```python
from build123d import *

# Parameters (mm, degrees)
SKETCH_1_R               = 4.9
EXTRUDE_1_DEPTH          = 1.5
SKETCH_3_R               = 3.9
EXTRUDE_2_DEPTH          = 3
SKETCH_4_R               = 4.9
EXTRUDE_3_DEPTH          = 1.3
CUT_EXTRUDE_1_DEPTH      = 10.036592278
CUT_EXTRUDE_1_DEPTH_BACK = 10.036592278
SKETCH_6_R               = 0.5
CUT_EXTRUDE_2_DEPTH      = 10.036592278


with BuildPart() as part:
    # Эскиз1 → Бобышка-Вытянуть1 (new body)
    with BuildSketch(Plane.XY):
        Circle(SKETCH_1_R)
    extrude(amount=EXTRUDE_1_DEPTH)

    # Эскиз3 → Бобышка-Вытянуть2 (add)
    with BuildSketch(Plane.XY.offset(1.5)):
        Circle(SKETCH_3_R)
    extrude(amount=EXTRUDE_2_DEPTH)

    # Эскиз4 → Бобышка-Вытянуть3 (add)
    with BuildSketch(Plane.XY.offset(4.5)):
        Circle(SKETCH_4_R)
    extrude(amount=EXTRUDE_3_DEPTH)

    # Эскиз5 → Вырез-Вытянуть1 (cut, two sides: drawn at the far end of the back side and taken through both)
    with BuildSketch(Plane(origin=(0, 0, 0), x_dir=(1, 0, 0), z_dir=(0, 1, 0)).offset(-CUT_EXTRUDE_1_DEPTH_BACK)):
        Polygon((1.45, 0), (0.971990262, -0.75), (-0.971990262, -0.75), (-1.45, 0), (-1.45, 0.521018793), (1.45, 0.521018793), align=None)
    extrude(amount=CUT_EXTRUDE_1_DEPTH + CUT_EXTRUDE_1_DEPTH_BACK, mode=Mode.SUBTRACT)

    # Эскиз6 → Вырез-Вытянуть2 (cut, through all)
    with BuildSketch(Plane.XY.offset(5.8)):
        with Locations((-4.9, 0)):
            Circle(SKETCH_6_R)
        with Locations((4.9, 0)):
            Circle(SKETCH_6_R)
    extrude(amount=-CUT_EXTRUDE_2_DEPTH, mode=Mode.SUBTRACT)


solid = part.part
```
Source: CAD feature listing. Evaluate the final solid. Frame: model axes, mm. A direction names the side the tool comes from. Round coordinates to 2 decimals unless told otherwise and drop trailing zeros. Loops run counter-clockwise (first coordinate to the right, second up) from the corner with the lowest first, then second, coordinate; pieces in that order, holes last.
(1) Material intervals for probe 1 along Z at (x, y) = (4, 0.5); probe 2 along Z at (x, y) = (0.5, -4); probe 3 along X at (y, z) = (3.75, 0.7), sorted ascending.
From the geometry:
probe 1: z = 0 to 1.5, 4.5 to 5.8
probe 2: z = 0.75 to 1.5, 4.5 to 5.8
probe 3: x = -3.15 to -1, 1 to 3.15
(2) Section query C-C (z = 0.4). Output: boundary loops of the cut face in (x, y), and give its area (3 significant figures).
From the geometry:
outline: (-4.87, -0.5) arc R4.9 ccw to (-1.2, -4.75) - (-1.2, 4.75) arc R4.9 ccw to (-4.87, 0.5) arc R0.5 cw to start; (1.2, -4.75) arc R4.9 ccw to (4.87, -0.5) arc R0.5 cw to (4.87, 0.5) arc R4.9 ccw to (1.2, 4.75) - close
area: 51.5 mm2
(3) Section query A-A (x = 0). Output: boundary loops of the cut face in (y, z), and give its area (3 significant figures).
From the geometry:
outline: (-4.9, 0.75) - (4.9, 0.75) - (4.9, 1.5) - (3.9, 1.5) - (3.9, 4.5) - (4.9, 4.5) - (4.9, 5.8) - (-4.9, 5.8) - (-4.9, 4.5) - (-3.9, 4.5) - (-3.9, 1.5) - (-4.9, 1.5) - close
area: 43.5 mm2
(4) Access query for faces 1 (the flat face through (0, 0, 0.75)), 2 (the flat face through (-4, -1, 4.5)), 3 (the cylindrical face through (-4.4, 0, 0.8)). Directions: +Z, -Z, +X, -X, +Y, -Y. A direction counts if a zero-diameter tool reaches every point of the face in a straight line with its end or side. Return the directions, or none.
From the geometry:
face 1: -Z, +Y, -Y
face 2: none
face 3: +Z, -Z, -X
(5) Pull-direction query (Z, two-part tool) for faces 4 (the flat face through (3, 0, 0)), 5 (the flat face through (-4, -1, 1.5)), 6 (the cylindrical face through (-0.1, -4.9, 5.1)); classes: +Z half, -Z half, draft (parallel to the pull), parting line (faces both ways), or undercut.
From the geometry:
face 4: -Z half
face 5: undercut
face 6: draft
(6) Contact query for flat-ended pins moving along their axis: pin 1 Ø1.6 at (x, y) = (0, -0.5) entering from -Z; pin 2 Ø1 at (x, z) = (3, 4.5) entering from -Y. Output: stop coordinate, or through.
From the geometry:
pin 1: stops at z = 0.75
pin 2: stops at y = -4.21
(7) Section query B-B (y = 0). Output: boundary loops of the cut face in (x, z).
From the geometry:
outline: (-4.4, 0) - (-1.45, 0) - (-0.97, 0.75) - (0.97, 0.75) - (1.45, 0) - (4.4, 0) - (4.4, 1.5) - (3.9, 1.5) - (3.9, 4.5) - (4.4, 4.5) - (4.4, 5.8) - (-4.4, 5.8) - (-4.4, 4.5) - (-3.9, 4.5) - (-3.9, 1.5) - (-4.4, 1.5) - close
